from build123d import *

# Parameters (mm, degrees)
SKETCH3_W                   = 0.5
SKETCH3_H                   = 2
LPATTERN1_COUNT             = 7
LPATTERN1_PITCH             = 5
M3_5X0_6_TAPPED_HOLE1_D     = 2.9
M3_5X0_6_TAPPED_HOLE1_DEPTH = 10
M3_5X0_6_TAPPED_HOLE1_TIP   = 0.871247898


with BuildPart() as part:
    # Sketch2 → Revolve1 (revolve)
    with BuildSketch(Plane.XY, mode=Mode.PRIVATE) as revolve1_sk:
        Polygon((0, 0), (-11.5, 0), (-11.5, -40), (-5.5, -40), (-5.5, -7), (0, -7), align=None)
    revolve(revolve1_sk.sketch.rotate(Axis((0, 0, 0), (0, -1, 0)), 270), axis=Axis((0, 0, 0), (0, -1, 0)))

    # Sketch3 → Cut-Revolve1 (revolve, cut)
    with BuildSketch(Plane.XY, mode=Mode.PRIVATE) as cut_revolve1_sk:
        with Locations((11.25, -36)):
            Rectangle(SKETCH3_W, SKETCH3_H)
    cut_revolve1 = revolve(cut_revolve1_sk.sketch.rotate(Axis((0, 0, 0), (0, -1, 0)), 90), axis=Axis((0, 0, 0), (0, -1, 0)), mode=Mode.SUBTRACT)

    # LPattern1: Cut-Revolve1 ×7
    with Locations(*[(0, i * LPATTERN1_PITCH, 0) for i in range(1, LPATTERN1_COUNT)]):
        add(cut_revolve1, mode=Mode.SUBTRACT)

    # M3.5x0.6 Tapped Hole1
    with Locations(Plane(origin=(0, 0, 0), x_dir=(1, 0, 0), z_dir=(0, 1, 0))):
        with Locations((8.5, 0), (0, 0), (-8.5, 0), (0, 8.5), (0, -8.5)):
            Hole(M3_5X0_6_TAPPED_HOLE1_D / 2, depth=M3_5X0_6_TAPPED_HOLE1_DEPTH)
            with Locations((0, 0, -(M3_5X0_6_TAPPED_HOLE1_DEPTH + M3_5X0_6_TAPPED_HOLE1_TIP / 2))):  # 118° drill point
                Cone(0, M3_5X0_6_TAPPED_HOLE1_D / 2, M3_5X0_6_TAPPED_HOLE1_TIP, mode=Mode.SUBTRACT)


solid = part.part
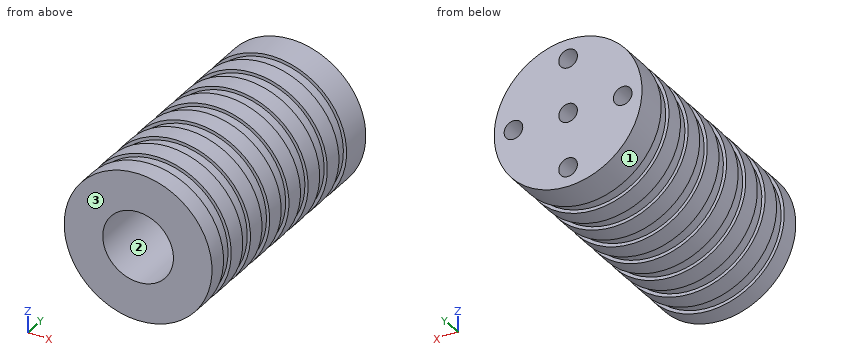
Can you work these out from the model? Positions are in its coordinate system, mm. Face numbers are marked on the shaded views. Round coordinates to 2 decimals unless told otherwise and drop trailing zeros. Loops run counter-clockwise (first coordinate to the right, second up) from the corner with the lowest first, then second, coordinate; pieces in that order, holes last. Notation, with made-up numbers: (83, -24.75) - (89, -24.75) arc R31 cw to (89, 2.25) - close; hole circle Ø6 at (3.25, -18). An arc over 180 degrees is marked (long way). Answer in a Markdown table with one row per item. Add a question column.
Q1. I want a section at B-B on y = -21.5. List the corners of the cut face in (x, z) for me, and give its area (3 significant figures).
Q2. I need wall thicknesses on L1, parallel to Y at x = 4.25, z = 0.5; L2, parallel to Z at x = 1.25, y = -28; L3, parallel to Z at x = -1, y = -31. Which ranges of each line are inside material? Lowest first, please.
Q3. We'd pull the mould along Z, two halves only. Please class the marked faces 1, 2 and 3: pulls with the +Z half, pulls with the -Z half, needs draft (parallel to the pull), parting line crosses it, or undercut.
Q4. For pin 1 Ø3.5 at (x, z) = (0, 1) entering from -Y; pin 2 Ø3 at (y, z) = (-22, 5) entering from +X; pin 3 Ø2 at (y, z) = (-5, -6) entering from -X, each with a flat end and sliding along its axis, tell me the tip position at first contact or that it passes through.
Q5. I want a section at A-A on y = -27.5. List the corners of the cut face in (x, z) for me.
A:
| question | item | result |
|---|---|---|
| 1 | outline | circle Ø22 at (0, 0); hole circle Ø11 at (0, 0) |
| 1 | area | 285 mm^2 |
| 2 | L1 | -7 to 0 |
| 2 | L2 | -11.43 to -5.36, 5.36 to 11.43 |
| 2 | L3 | -10.95 to -5.41, 5.41 to 10.95 |
| 3 | face 1 | parting line crosses it |
| 3 | face 2 | undercut |
| 3 | face 3 | needs draft |
| 4 | pin 1 | y = -7 |
| 4 | pin 2 | x = 10.95 |
| 4 | pin 3 | x = -10.36 |
| 5 | outline | circle Ø23 at (0, 0); hole circle Ø11 at (0, 0) |
